from build123d import *

# Parameters (mm, degrees)
F1_DEPTH = 3.175
F2_R     = 2.54
F3_R     = 2.54


with BuildPart() as f1:
    # F0 (on Front) → F1 (new body)
    with BuildSketch(Plane.XZ):
        with BuildLine():
            ThreePointArc((-257.224470377, -23.4096460044), (-230.192520377, -36.1096460044), (-203.160570377, -23.4096460044))
            ThreePointArc((-203.160570377, -23.4096460044), (-230.192520377, -10.7096460044), (-257.224470377, -23.4096460044))
        make_face()
    extrude(amount=F1_DEPTH)

    # F2
    f2_edges = [f1.edges().sort_by_distance(p)[0] for p in [
        (-203.16057, -1.5875, -23.409646),
    ]]
    fillet(f2_edges, radius=F2_R)

    # F3
    f3_edges = [f1.edges().sort_by_distance(p)[0] for p in [
        (-257.22447, -1.5875, -23.409646),
    ]]
    fillet(f3_edges, radius=F3_R)


solid = f1.part
Can you work these out from the model? Positions are in its coordinate system, mm. Coordinates: 2 decimals unless noted, no trailing zeros. Write each loop counter-clockwise with the first axis right and the second up, starting at its lowest first coordinate (ties: lowest second). Pieces come first, ordered by that corner, then holes. Notation, with made-up numbers: M 87,0.5 L 139,0.5 A10 cw 139,15.5 Z; hole C 55.25,50.25 d4. An arc over 180 degrees is marked long. Use one line per item in the form item = value.
Q1. If we section it at A-A (z = -28): Write out the boundary of the cut face in (x, y) (3 decimals), then the cut area to 3 significant figures.
Model answer:
outline = M -252.639,-3.175 L -207.746,-3.175 L -207.746,0 L -252.639,0 Z
area = 143 mm^2
Q2. If we section it at B-B (x = -224): Write out the boundary of the cut face in (y, z) (3 decimals).
Model answer:
outline = M -3.175,-35.559 L 0,-35.559 L 0,-11.26 L -3.175,-11.26 Z
Q3. I need wall thicknesses on line 1 along Z through (x, y) = (-220, -0.55); line 2 along Z through (x, y) = (-237, -1.6); line 3 along X through (y, z) = (-1.05, -20). Which ranges of each line are inside material? Lowest first, please. Write a range as from..to.
Model answer:
line_1 = -34.6..-12.22
line_2 = -35.44..-11.38
line_3 = -253.99..-206.4
